Geometry: final body of the model. Coordinates: model frame, mm. Give positions to 0.01 mm unless a question says otherwise; leave off trailing zeros. Order: outer loops, then holes, each group sorted by start corner. A loop starts at its lowest first (then second) coordinate and runs counter-clockwise, first axis right, second up. Notation, with made-up numbers: (44, 84.5) -> (57, 84.5) arc R13 ccw to (57, 97.5) -> close; hole circle Ø3 at (4.5, 54). An arc over 180 degrees is marked (long way). One line per question, with ' | ' between items. Start each with the question number.
(1) Section D-D (z = 35). Return loops of the section in (x, y), then the cut area to 3 significant figures.
(2) First-contact query: pin 1 Ø1 at (y, z) = (0.5, -9) entering from +X. Flat tip, straight axial feed; report the tip coordinate or a pass-through.
(3) Ray query, L1, parallel to Z at x = 0, y = 2.3; L2, parallel to X at y = 0.9, z = 35; L3, parallel to X at y = 1.55, z = -23. Return the intervals inside material, ascending.
(4) Section C-C (y = 0.5). Return loops of the section in (x, z).
(5) Mould query, pull axis Z, two halves, no side actions, for faces 1 (the face through (1, 3, -8)), 2 (the face through (-0.07, 1.48, 33.4)), 3 (the face through (-0.867, 1.521, 3.905)), 4 (the face through (8.67, 1.48, 39.05)). Classes: +Z half, -Z half, draft (parallel to the pull), parting line (faces both ways), or undercut.
(6) Section A-A (x = 0). Return loops of the section in (y, z), then the cut area to 3 significant figures.
(7) Section B-B (z = 0). Return loops of the section in (x, y), then the cut area to 3 significant figures.
Autodesk Inventor part; units mm, degrees
ref_plane "YZ Plane" through (0, 0, 0) normal (1, 0, 0) x (0, 1, 0)
ref_plane "XZ Plane" through (0, 0, 0) normal (0, 1, 0) x (-1, 0, 0)
ref_plane "XY Plane" through (0, 0, 0) normal (0, 0, 1) x (1, 0, 0)
sketch "スケッチ1" plane through (0, 0, 0) normal (0, 1, 0) x (-1, 0, 0)
  circle A0 centre (0, 0) radius 40
  dimension "d0" = 80
extrude "押し出し1" add sketch "スケッチ1" along normal blind 3
sketch "スケッチ2" plane through (0, 3, 0) normal (0, 1, 0) x (1, 0, 0)
  circle A0 centre (0, 0) radius 4
  dimension "d3" = 8
extrude "押し出し2" cut sketch "スケッチ2" against normal blind 3
sketch "スケッチ3" plane through (0, 3, 0) normal (0, 1, 0) x (1, 0, 0)
  circle A0 centre (0, -35) radius 1.6
  circle A1 centre (0, 0) radius 40
  dimension "d6" = 3.2
  dimension "d7" = 35
hole "穴1" at (0, 3, 35) direction (0, -1, 0) diameter 3.2 end through all
properties part number "NHK_t0_2"
Response:
1) outline: (-19.36, 0) -> (-1.6, 0) -> (-1.6, 3) -> (-19.36, 3) -> close; (1.6, 0) -> (19.36, 0) -> (19.36, 3) -> (1.6, 3) -> close | area: 107 mm^2
2) pin 1: stops at x = 39.09
3) L1: z = -40 to -4, 4 to 33.4, 36.6 to 40 | L2: x = -19.36 to -1.6, 1.6 to 19.36 | L3: x = -32.73 to 32.73
4) outline: circle Ø80 at (0, 0); hole circle Ø8 at (0, 0); hole circle Ø3.2 at (0, 35)
5) face 1: draft | face 2: undercut | face 3: undercut | face 4: parting line
6) outline: (0, -40) -> (3, -40) -> (3, -4) -> (0, -4) -> close; (0, 4) -> (3, 4) -> (3, 33.4) -> (0, 33.4) -> close; (0, 36.6) -> (3, 36.6) -> (3, 40) -> (0, 40) -> close | area: 206 mm^2
7) outline: (-40, 0) -> (-4, 0) -> (-4, 3) -> (-40, 3) -> close; (4, 0) -> (40, 0) -> (40, 3) -> (4, 3) -> close | area: 216 mm^2
